The drawing under review shows one solid part. Ordinate dimensions are in mm from its lowest x, y, z. Coordinates: 2 decimals unless noted, no trailing zeros. Write each loop counter-clockwise with the first axis right and the second up, starting at its lowest first coordinate (ties: lowest second). Pieces come first, ordered by that corner, then holes.
1) For P1, Ø1.5, axis at y = 19, z = 2, coming from the -X side; P2, Ø1.5, axis at x = 7, y = 11.5, coming from the +Z side; P3, Ø1, axis at y = 19.5, z = 3.5, coming from the +X side; P4, Ø1.5, axis at y = 2.5, z = 10, coming from the +X side, all flat-tipped, find the tip position at first contact; note any pin that passes through.
2) Add section A-A, the plane z = 7.5. State the section outline as (x, y) points, then the cut area to 3 significant figures.
3) For line 1 (Z direction, x = 7.5, y = 5.5); line 2 (Z direction, x = 5.75, y = 1.25), list the stretches that pass through material, from the lowest coordinate up.
4) Mouldability with a two-part tool opening along X and no side actions: class the marked faces 1, 2 and 3 as released by +X, released by -X, zero draft, split by the parting line, or undercut.
5) Add section C-C, the plane y = 11.25. State the section outline as (x, z) points.
6) Add section B-B, the plane x = 7.5. State the section outline as (y, z) points, then the cut area to 3 significant figures.
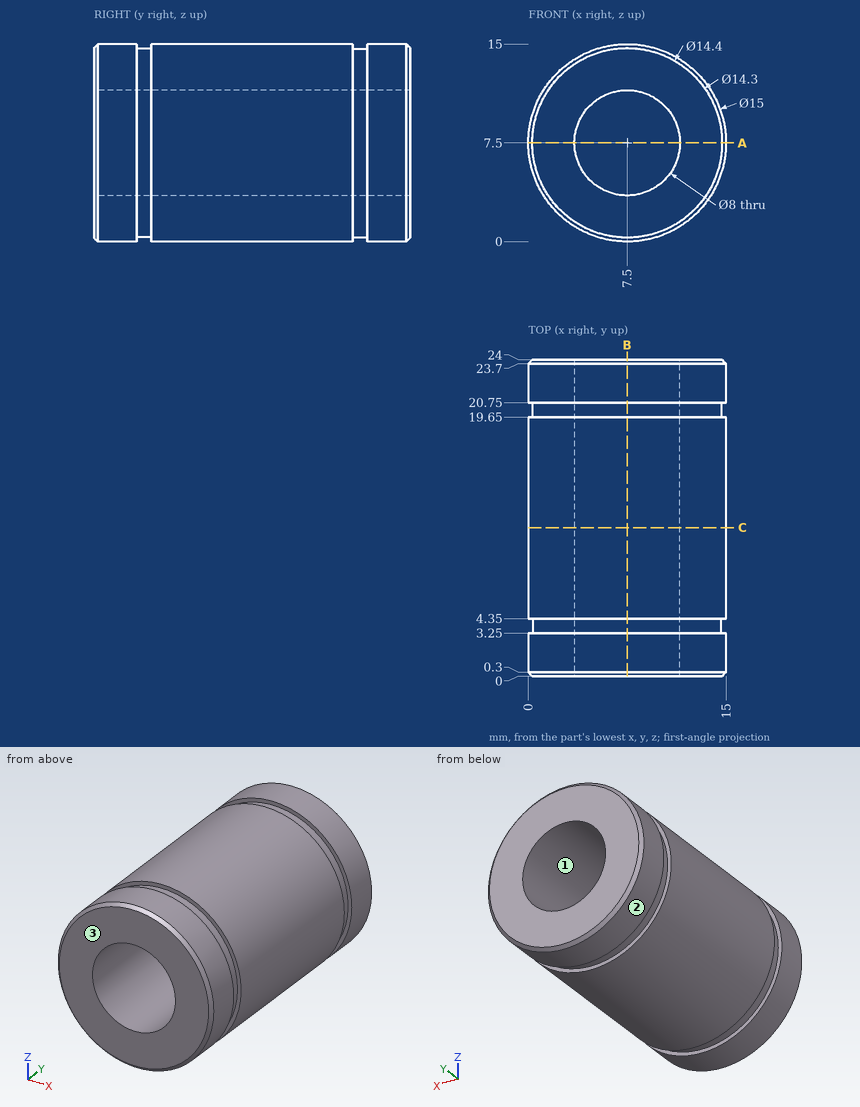
Geometry results:
1. P1: stops at x = 1.7
1. P2: stops at z = 15
1. P3: stops at x = 14.13
1. P4: stops at x = 14.79
2. outline: (0, 0.3) - (0.3, 0) - (3.5, 0) - (3.5, 24) - (0.3, 24) - (0, 23.7) - (0, 20.75) - (0.35, 20.75) - (0.35, 19.65) - (0, 19.65) - (0, 4.35) - (0.35, 4.35) - (0.35, 3.25) - (0, 3.25) - close; (11.5, 0) - (14.7, 0) - (15, 0.3) - (15, 3.25) - (14.65, 3.25) - (14.65, 4.35) - (15, 4.35) - (15, 19.65) - (14.65, 19.65) - (14.65, 20.75) - (15, 20.75) - (15, 23.7) - (14.7, 24) - (11.5, 24) - close
2. area: 166 mm2
3. line 1: z = 0 to 3.5, 11.5 to 15
3. line 2: z = 0.21 to 3.9, 11.1 to 14.79
4. face 1: undercut
4. face 2: split by the parting line
4. face 3: zero draft
5. outline: circle Ø15 at (7.5, 7.5); hole circle Ø8 at (7.5, 7.5)
6. outline: (0, 0.3) - (0.3, 0) - (3.25, 0) - (3.25, 0.35) - (4.35, 0.35) - (4.35, 0) - (19.65, 0) - (19.65, 0.35) - (20.75, 0.35) - (20.75, 0) - (23.7, 0) - (24, 0.3) - (24, 3.5) - (0, 3.5) - close; (0, 11.5) - (24, 11.5) - (24, 14.7) - (23.7, 15) - (20.75, 15) - (20.75, 14.65) - (19.65, 14.65) - (19.65, 15) - (4.35, 15) - (4.35, 14.65) - (3.25, 14.65) - (3.25, 15) - (0.3, 15) - (0, 14.7) - close
6. area: 166 mm2
